from build123d import *

# Parameters (mm, degrees)
CROQUIS1_W              = 4.8
CROQUIS1_H              = 2.4
CROQUIS1_W_2            = 22.5
CROQUIS1_H_2            = 23.8
SALIENTE_EXTRUIR1_DEPTH = 6.2
SALIENTE_EXTRUIR2_DEPTH = 4.2
CORTAR_EXTRUIR1_REACH   = 21.5
CORTAR_EXTRUIR3_DEPTH   = 0.8
CROQUIS4_5_W            = 1.5
CROQUIS4_5_H            = 3.75
CORTAR_EXTRUIR4_DEPTH   = 2
CORTAR_EXTRUIR5_DEPTH   = 13.4
CROQUIS7_R              = 2.425
CROQUIS7_R_2            = 0.875
SALIENTE_EXTRUIR4_DEPTH = 2.85


with BuildPart() as part:
    # Croquis1 → Saliente-Extruir1 (new body, symmetric)
    with BuildSketch(Plane.XY):
        with Locations((-13.65, 6.4)):
            Rectangle(CROQUIS1_W, CROQUIS1_H)
        Rectangle(CROQUIS1_W_2, CROQUIS1_H_2)
        with Locations((13.65, 6.4)):
            Rectangle(CROQUIS1_W, CROQUIS1_H)
    extrude(amount=SALIENTE_EXTRUIR1_DEPTH, both=True)

    # Croquis2 → Saliente-Extruir2 (add)
    with BuildSketch(Plane(origin=(0, 11.9, 0), x_dir=(1, 0, 0), z_dir=(0, 1, 0))):
        with BuildLine():
            ThreePointArc((-0.484210526, -2.79508745), (11.25, 0), (-0.484210526, 2.79508745))
            ThreePointArc((-0.484210526, 2.79508745), (-3.45, 0), (-0.484210526, -2.79508745))
        make_face()
    extrude(amount=SALIENTE_EXTRUIR2_DEPTH)

    # Croquis3 → Cortar-Extruir1 (cut, up to next)
    with BuildSketch(Plane(origin=(0, 7.6, 0), x_dir=(1, 0, 0), z_dir=(0, 1, 0)), mode=Mode.PRIVATE) as cortar_extruir1_sk1:
        with BuildLine():
            Line((16.05, 0.575), (14.815922382, 0.575))
            ThreePointArc((14.815922382, 0.575), (12.35, 0), (14.815922382, -0.575))
            Line((14.815922382, -0.575), (16.05, -0.575))
            Line((16.05, -0.575), (16.05, 0.575))
        make_face()
    cortar_extruir1_tool1 = extrude(cortar_extruir1_sk1.sketch, amount=-CORTAR_EXTRUIR1_REACH, mode=Mode.PRIVATE) & part.part
    add(cortar_extruir1_tool1.solids().sort_by_distance((14.012834, 7.6, 0))[0], mode=Mode.SUBTRACT)
    # Croquis3 → Cortar-Extruir1 (cut, up to next)
    with BuildSketch(Plane(origin=(0, 7.6, 0), x_dir=(1, 0, 0), z_dir=(0, 1, 0)), mode=Mode.PRIVATE) as cortar_extruir1_sk2:
        with BuildLine():
            Line((-16.05, 0.575), (-14.815922382, 0.575))
            ThreePointArc((-14.815922382, 0.575), (-12.35, 0), (-14.815922382, -0.575))
            Line((-14.815922382, -0.575), (-16.05, -0.575))
            Line((-16.05, -0.575), (-16.05, 0.575))
        make_face()
    cortar_extruir1_tool2 = extrude(cortar_extruir1_sk2.sketch, amount=-CORTAR_EXTRUIR1_REACH, mode=Mode.PRIVATE) & part.part
    add(cortar_extruir1_tool2.solids().sort_by_distance((-14.012834, 7.6, 0))[0], mode=Mode.SUBTRACT)

    # Croquis4 → Cortar-Extruir3 (cut)
    with BuildSketch(Plane.XZ.offset(11.9)):
        with BuildLine():
            Line((-11.25, 6.2), (-11.25, 3.3))
            ThreePointArc((-11.25, 3.3), (-9.199390335, 4.149390335), (-8.35, 6.2))
            Line((-8.35, 6.2), (-11.25, 6.2))
        make_face()
        with BuildLine():
            ThreePointArc((-8.35, -6.2), (-9.199390335, -4.149390335), (-11.25, -3.3))
            Line((-11.25, -3.3), (-11.25, -6.2))
            Line((-11.25, -6.2), (-8.35, -6.2))
        make_face()
    extrude(amount=-CORTAR_EXTRUIR3_DEPTH, mode=Mode.SUBTRACT)

    # Croquis4_5 → Cortar-Extruir4 (cut)
    with BuildSketch(Plane.XZ.offset(11.9)):
        with BuildLine():
            Line((11.25, 6.2), (8.35, 6.2))
            ThreePointArc((8.35, 6.2), (9.199390335, 4.149390335), (11.25, 3.3))
            Line((11.25, 3.3), (11.25, 6.2))
        make_face()
        with BuildLine():
            ThreePointArc((11.25, -3.3), (9.199390335, -4.149390335), (8.35, -6.2))
            Line((8.35, -6.2), (11.25, -6.2))
            Line((11.25, -6.2), (11.25, -3.3))
        make_face()
        with Locations((10.5, 0)):
            Rectangle(CROQUIS4_5_W, CROQUIS4_5_H)
    extrude(amount=-CORTAR_EXTRUIR4_DEPTH, mode=Mode.SUBTRACT)

    # Croquis6 → Cortar-Extruir5 (cut, through all)
    with BuildSketch(Plane(origin=(0, 0, -6.2), x_dir=(-1, 0, 0), z_dir=(0, 0, -1))):
        Polygon((-11.25, -9.9), (-8.35, -11.9), (-11.25, -11.9), align=None)
    extrude(amount=-CORTAR_EXTRUIR5_DEPTH, mode=Mode.SUBTRACT)

    # Croquis7 → Saliente-Extruir4 (add)
    with BuildSketch(Plane(origin=(0, 16.1, 0), x_dir=(1, 0, 0), z_dir=(0, 1, 0))):
        with Locations((5.05, 0)):
            Circle(CROQUIS7_R)
        with Locations((5.05, 0)):
            Circle(CROQUIS7_R_2, mode=Mode.SUBTRACT)
    extrude(amount=SALIENTE_EXTRUIR4_DEPTH)


solid = part.part
The model under review builds one solid part; all positions refer to its coordinate system, in mm. A direction names the side the tool comes from. Coordinates: 2 decimals unless noted, no trailing zeros. Write each loop counter-clockwise with the first axis right and the second up, starting at its lowest first coordinate (ties: lowest second). Pieces come first, ordered by that corner, then holes. Notation, with made-up numbers: (19.25, -30) -> (49.25, -30) arc R23 cw to (49.25, -7) -> close; hole circle Ø5 at (-14, 6). An arc over 180 degrees is marked (long way). Answer in a Markdown table with one row per item.
1. Draft analysis for pull direction Z (two halves, no side actions). For faces 6 (the cylindrical face through (-12.35, 6.42, -0.05)), 7 (the flat face through (-2, -11.9, 0)), 8 (the flat face through (10.2, -10.2, -1.875)), 9 (the cylindrical face through (8.9, -10.7, -4.5)), state which applies: +Z half, -Z half, draft (parallel to the pull), parting line (faces both ways), or undercut.
Answers below:
| item | result |
|---|---|
| face 6 | undercut |
| face 7 | draft |
| face 8 | undercut |
| face 9 | -Z half |
2. We need section B-B, the plane z = 4.75. State the section outline as (x, y) points, and give its area (3 significant figures).
Answers below:
| item | result |
|---|---|
| outline | (-16.05, 5.2) -> (-11.25, 5.2) -> (-11.25, -11.1) -> (-8.74, -11.1) -> (-8.74, -11.9) -> (8.35, -11.9) -> (8.74, -11.63) -> (8.74, -9.9) -> (11.25, -9.9) -> (11.25, 5.2) -> (16.05, 5.2) -> (16.05, 7.6) -> (11.25, 7.6) -> (11.25, 11.9) -> (9.03, 11.9) -> (9.03, 16.1) -> (1.07, 16.1) -> (1.07, 11.9) -> (-11.25, 11.9) -> (-11.25, 7.6) -> (-16.05, 7.6) -> close |
| area | 585 mm^2 |
3. Clearance check with flat-ended pins moving along their axes: pin 1 Ø2 at (x, z) = (-6.5, -1) entering from +Y; pin 2 Ø1.9 at (x, z) = (9, -4) entering from +Y; pin 3 Ø1.5 at (x, z) = (9, 4) entering from -Y; pin 4 Ø4 at (x, z) = (14.5, 3) entering from +Y. State where each tip first meets the part, or that it passes through.
Answers below:
| item | result |
|---|---|
| pin 1 | stops at y = 11.9 |
| pin 2 | stops at y = 16.1 |
| pin 3 | stops at y = -11.9 |
| pin 4 | stops at y = 7.6 |
4. For faces 1 (the flat face through (10, -9.9, -5)), 2 (the flat face through (13.6, 5.2, 1.5)), 3 (the cylindrical face through (-9.18, -11.51, -4.17)), 4 (the cylindrical face through (7.3, 17.5, 0.9)), 5 (the flat face through (-10, -11.1, 5)), list the 3-axis set-ups (+Z, -Z, +X, -X, +Y, -Y) from which the entire face can be reached by the end or side of a thin tool; tool diameter is ignored.
Answers below:
| item | result |
|---|---|
| face 1 | -Z, +X, -Y |
| face 2 | +Z, -Z, +X, -Y |
| face 3 | -Z, -X, -Y |
| face 4 | +Y |
| face 5 | +Z, -X, -Y |
5. We need section C-C, the plane x = -4. State the section outline as (y, z) points, and give its area (3 significant figures).
Answers below:
| item | result |
|---|---|
| outline | (-11.9, -6.2) -> (11.9, -6.2) -> (11.9, 6.2) -> (-11.9, 6.2) -> close |
| area | 295 mm^2 |
6. We need section D-D, the plane y = -7. State the section outline as (x, z) points, and give its area (3 significant figures).
Answers below:
| item | result |
|---|---|
| outline | (-11.25, -6.2) -> (11.25, -6.2) -> (11.25, 6.2) -> (-11.25, 6.2) -> close |
| area | 279 mm^2 |
7. We need section A-A, the plane x = 13.65. State the section outline as (y, z) points, and give its area (3 significant figures).
Answers below:
| item | result |
|---|---|
| outline | (5.2, -6.2) -> (7.6, -6.2) -> (7.6, -1.3) -> (5.2, -1.3) -> close; (5.2, 1.3) -> (7.6, 1.3) -> (7.6, 6.2) -> (5.2, 6.2) -> close |
| area | 23.5 mm^2 |
8. Wall thickness on probe 1 along Z at (x, y) = (5.05, 17.95) (3 decimals); probe 2 along Z at (x, y) = (13.65, 7); probe 3 along Y at (x, z) = (13, 1.5): over which ranges is each line inside the solid? List them lowest first. Write a range as [from, to].
Answers below:
| item | result |
|---|---|
| probe 1 | z = [-2.425, -0.875], [0.875, 2.425] |
| probe 2 | z = [-6.2, -1.3], [1.3, 6.2] |
| probe 3 | y = [5.2, 7.6] |
